Here's how the part is built. I have some questions about the finished solid (model axes, mm). Coordinates: 2 decimals unless noted, no trailing zeros. Loops run counter-clockwise (first coordinate to the right, second up) from the corner with the lowest first, then second, coordinate; pieces in that order, holes last. Notation, with made-up numbers: (12.5, 20.25) -> (51.5, 20.25) arc R31 cw to (51.5, 56.25) -> close; hole circle Ø6 at (61, 78). An arc over 180 degrees is marked (long way). Answer as a JSON object with one key per item and string values. Group by question number.
Q1. I want a section at B-B on x = 152. Write out the boundary of the cut face in (y, z).
Q2. I need wall thicknesses on line 1 (Z direction, x = 373, y = -265); line 2 (Z direction, x = 249, y = -689). Which ranges of each line are inside material? Lowest first, please.
Q3. Thinking about a two-plate mould opening in X: for faces 1 (the cylindrical face through (683.7, -591.6, 17.2)), 2 (the cylindrical face through (455.7, -591.6, 17.2)), which applies, released by +X, released by -X, zero draft, split by the parting line, or undercut?
Q4. I want a section at A-A on z = 14. Count the separate pieces of the cut face and the enclosed holes in it, then the cut area to 3 significant figures.
Q5. I'm going to push flat-ended pins straight in: pin 1 (4 mm diameter, centred on y = -459.5, z = 13, fed in from -X); pin 2 (6 mm diameter, centred on x = 667.5, y = -290.5, fed in from +Z); pin 3 (1.5 mm diameter, centred on x = 206, y = -341, fed in from -Z). Where does each tip first touch, or does it pass through?
```python
from build123d import *

# Parameters (mm, degrees)
F1_DEPTH = 1200


with BuildPart() as f1:
    # F0 (on Front) → F1 (new body)
    with BuildSketch(Plane.XZ):
        with BuildLine():
            ThreePointArc((38, 0), (27.488102, 2.363771), (19, 9))
            ThreePointArc((19, 9), (0, 18), (-19, 9))
            ThreePointArc((-19, 9), (-27.488102, 2.363771), (-38, 0))
            Line((-38, 0), (-38, -0.8))
            ThreePointArc((-38, -0.8), (-27.145633, 1.640781), (-18.380995, 8.493213))
            ThreePointArc((-18.380995, 8.493213), (0, 17.2), (18.380995, 8.493213))
            ThreePointArc((18.380995, 8.493213), (27.145633, 1.640781), (38, -0.8))
            ThreePointArc((38, -0.8), (48.854367, 1.640781), (57.619005, 8.493213))
            ThreePointArc((57.619005, 8.493213), (76, 17.2), (94.380995, 8.493213))
            ThreePointArc((94.380995, 8.493213), (103.145633, 1.640781), (114, -0.8))
            ThreePointArc((114, -0.8), (124.854367, 1.640781), (133.619005, 8.493213))
            ThreePointArc((133.619005, 8.493213), (152, 17.2), (170.380995, 8.493213))
            ThreePointArc((170.380995, 8.493213), (179.145633, 1.640781), (190, -0.8))
            ThreePointArc((190, -0.8), (200.854367, 1.640781), (209.619005, 8.493213))
            ThreePointArc((209.619005, 8.493213), (228, 17.2), (246.380995, 8.493213))
            ThreePointArc((246.380995, 8.493213), (255.145633, 1.640781), (266, -0.8))
            ThreePointArc((266, -0.8), (276.854367, 1.640781), (285.619005, 8.493213))
            ThreePointArc((285.619005, 8.493213), (304, 17.2), (322.380995, 8.493213))
            ThreePointArc((322.380995, 8.493213), (331.145633, 1.640781), (342, -0.8))
            ThreePointArc((342, -0.8), (352.854367, 1.640781), (361.619005, 8.493213))
            ThreePointArc((361.619005, 8.493213), (380, 17.2), (398.380995, 8.493213))
            ThreePointArc((398.380995, 8.493213), (407.145633, 1.640781), (418, -0.8))
            ThreePointArc((418, -0.8), (428.854367, 1.640781), (437.619005, 8.493213))
            ThreePointArc((437.619005, 8.493213), (456, 17.2), (474.380995, 8.493213))
            ThreePointArc((474.380995, 8.493213), (483.145633, 1.640781), (494, -0.8))
            ThreePointArc((494, -0.8), (504.854367, 1.640781), (513.619005, 8.493213))
            ThreePointArc((513.619005, 8.493213), (532, 17.2), (550.380995, 8.493213))
            ThreePointArc((550.380995, 8.493213), (559.145633, 1.640781), (570, -0.8))
            ThreePointArc((570, -0.8), (580.854367, 1.640781), (589.619005, 8.493213))
            ThreePointArc((589.619005, 8.493213), (608, 17.2), (626.380995, 8.493213))
            ThreePointArc((626.380995, 8.493213), (635.145633, 1.640781), (646, -0.8))
            ThreePointArc((646, -0.8), (656.854367, 1.640781), (665.619005, 8.493213))
            ThreePointArc((665.619005, 8.493213), (684, 17.2), (702.380995, 8.493213))
            ThreePointArc((702.380995, 8.493213), (711.145633, 1.640781), (722, -0.8))
            ThreePointArc((722, -0.8), (732.854367, 1.640781), (741.619005, 8.493213))
            ThreePointArc((741.619005, 8.493213), (760, 17.2), (778.380995, 8.493213))
            ThreePointArc((778.380995, 8.493213), (787.145633, 1.640781), (798, -0.8))
            Line((798, -0.8), (798, 0))
            ThreePointArc((798, 0), (787.488102, 2.363771), (779, 9))
            ThreePointArc((779, 9), (760, 18), (741, 9))
            ThreePointArc((741, 9), (732.511898, 2.363771), (722, 0))
            ThreePointArc((722, 0), (711.488102, 2.363771), (703, 9))
            ThreePointArc((703, 9), (684, 18), (665, 9))
            ThreePointArc((665, 9), (656.511898, 2.363771), (646, 0))
            ThreePointArc((646, 0), (635.488102, 2.363771), (627, 9))
            ThreePointArc((627, 9), (608, 18), (589, 9))
            ThreePointArc((589, 9), (580.511898, 2.363771), (570, 0))
            ThreePointArc((570, 0), (559.488102, 2.363771), (551, 9))
            ThreePointArc((551, 9), (532, 18), (513, 9))
            ThreePointArc((513, 9), (504.511898, 2.363771), (494, 0))
            ThreePointArc((494, 0), (483.488102, 2.363771), (475, 9))
            ThreePointArc((475, 9), (456, 18), (437, 9))
            ThreePointArc((437, 9), (428.511898, 2.363771), (418, 0))
            ThreePointArc((418, 0), (407.488102, 2.363771), (399, 9))
            ThreePointArc((399, 9), (380, 18), (361, 9))
            ThreePointArc((361, 9), (352.511898, 2.363771), (342, 0))
            ThreePointArc((342, 0), (331.488102, 2.363771), (323, 9))
            ThreePointArc((323, 9), (304, 18), (285, 9))
            ThreePointArc((285, 9), (276.511898, 2.363771), (266, 0))
            ThreePointArc((266, 0), (255.488102, 2.363771), (247, 9))
            ThreePointArc((247, 9), (228, 18), (209, 9))
            ThreePointArc((209, 9), (200.511898, 2.363771), (190, 0))
            ThreePointArc((190, 0), (179.488102, 2.363771), (171, 9))
            ThreePointArc((171, 9), (152, 18), (133, 9))
            ThreePointArc((133, 9), (124.511898, 2.363771), (114, 0))
            ThreePointArc((114, 0), (103.488102, 2.363771), (95, 9))
            ThreePointArc((95, 9), (76, 18), (57, 9))
            ThreePointArc((57, 9), (48.511898, 2.363771), (38, 0))
        make_face()
    extrude(amount=F1_DEPTH)


solid = f1.part
```
Result set:
{
 "1": {"outline": "(-1200, 17.2) -> (0, 17.2) -> (0, 18) -> (-1200, 18) -> close"},
 "2": {"line 1": "z = 16.15 to 16.98", "line 2": "z = 5.74 to 6.84"},
 "3": {"face 1": "undercut", "face 2": "undercut"},
 "4": {"separate pieces": "22", "enclosed holes": "0", "area": "40,300 mm²"},
 "5": {"pin 1": "stops at x = -17.17", "pin 2": "stops at z = 13.96", "pin 3": "stops at z = 4.3"}
}
